Input: dimensioned drawing with shaded views. Units: mm. Origin: part minimum x, y, z. A direction names the side the tool comes from. Round coordinates to 2 decimals unless told otherwise and drop trailing zeros. Loops run counter-clockwise (first coordinate to the right, second up) from the corner with the lowest first, then second, coordinate; pieces in that order, holes last. Notation, with made-up numbers: (5.25, 79.25) - (14.25, 79.25) arc R31 ccw to (14.25, 110.25) - close; hole circle Ø5 at (-32, -5.5). An arc over 180 degrees is marked (long way). Answer as CSV lines item,"result".
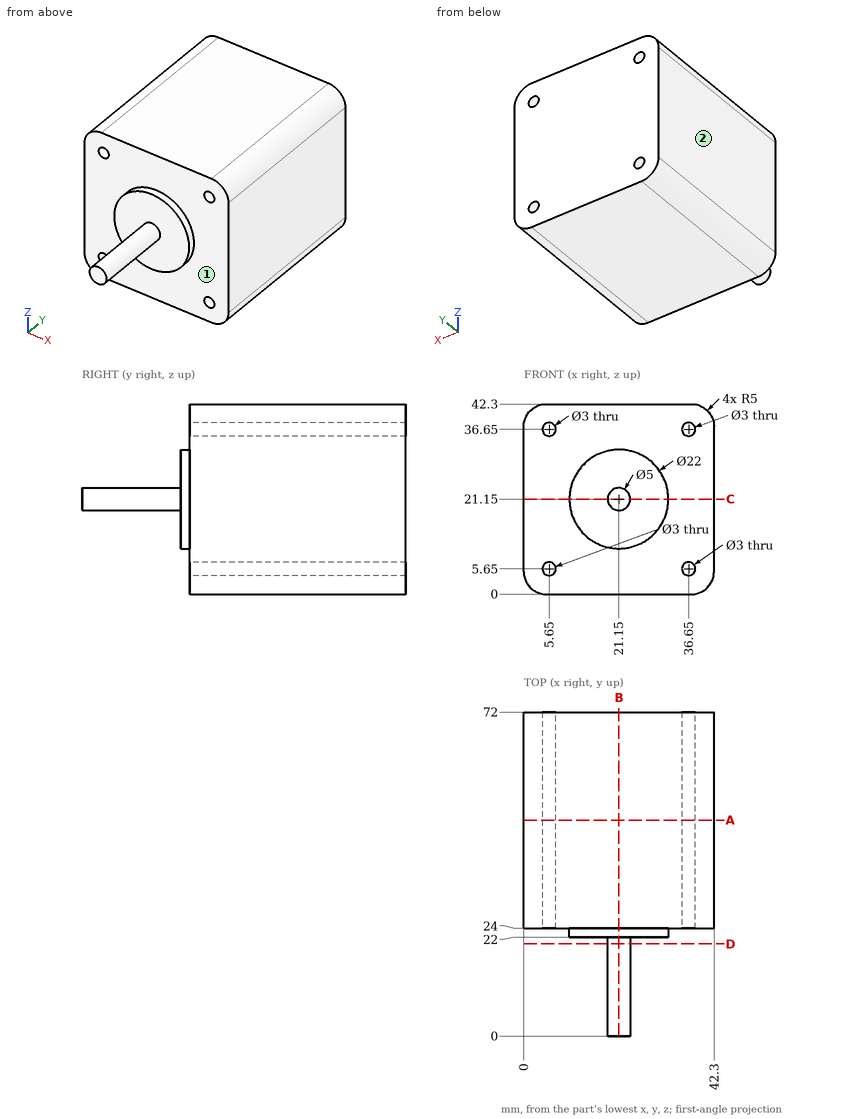
(1) Section D-D (y = 20.5). Output: boundary loops of the cut face in (x, z), and give its area (3 significant figures).
Findings below:
outline,"circle Ø5 at (21.15, 21.15)"
area,"19.6 mm2"
(2) Pin query (flat end, axial travel): P1, Ø4, axis at x = 36.65, z = 5.65, coming from the -Y side. Return the tip coordinate at first contact, or that it passes through.
Findings below:
P1,"y = 24"
(3) Material intervals for line 1 along Z through (x, y) = (36.65, 60); line 2 along X through (y, z) = (51, 36); line 3 along Y through (x, z) = (33, 32), sorted ascending.
Findings below:
line 1,"0 to 4.15, 7.15 to 35.15, 38.15 to 42.3"
line 2,"0 to 4.3, 7 to 35.3, 38 to 42.3"
line 3,"24 to 72"
(4) Section C-C (z = 21.15). Output: boundary loops of the cut face in (x, y).
Findings below:
outline,"(0, 24) - (10.15, 24) - (10.15, 22) - (18.65, 22) - (18.65, 0) - (23.65, 0) - (23.65, 22) - (32.15, 22) - (32.15, 24) - (42.3, 24) - (42.3, 72) - (0, 72) - close"
(5) Section B-B (x = 21.15). Output: boundary loops of the cut face in (y, z).
Findings below:
outline,"(0, 18.65) - (22, 18.65) - (22, 10.15) - (24, 10.15) - (24, 0) - (72, 0) - (72, 42.3) - (24, 42.3) - (24, 32.15) - (22, 32.15) - (22, 23.65) - (0, 23.65) - close"
(6) Access query for the marked faces 1 and 2. Directions: +Z, -Z, +X, -X, +Y, -Y. A direction counts if a zero-diameter tool reaches every point of the face in a straight line with its end or side. Return the directions, or none.
Findings below:
face 1,"-Y"
face 2,"+Z, -Z, -X, +Y, -Y"
(7) Section A-A (y = 48). Output: boundary loops of the cut face in (x, z), and give its area (3 significant figures).
Findings below:
outline,"(0, 5) arc R5 ccw to (5, 0) - (37.3, 0) arc R5 ccw to (42.3, 5) - (42.3, 37.3) arc R5 ccw to (37.3, 42.3) - (5, 42.3) arc R5 ccw to (0, 37.3) - close; hole circle Ø3 at (5.65, 5.65); hole circle Ø3 at (5.65, 36.65); hole circle Ø3 at (36.65, 5.65); hole circle Ø3 at (36.65, 36.65)"
area,"1,740 mm2"
